CAD build for the part. Positions are in the model's coordinates, mm. Face numbers are marked on the shaded views. A direction names the side the tool comes from. Give positions to 0.01 mm unless a question says otherwise; leave off trailing zeros. Write each loop counter-clockwise with the first axis right and the second up, starting at its lowest first coordinate (ties: lowest second). Pieces come first, ordered by that corner, then holes. Notation, with made-up numbers: (-8, 51.5) - (0, 51.5) arc R35 cw to (0, 84.5) - close; hole circle Ø8 at (82.25, 52.25). An arc over 180 degrees is marked (long way). Answer as a JSON object with one key per item and string values.
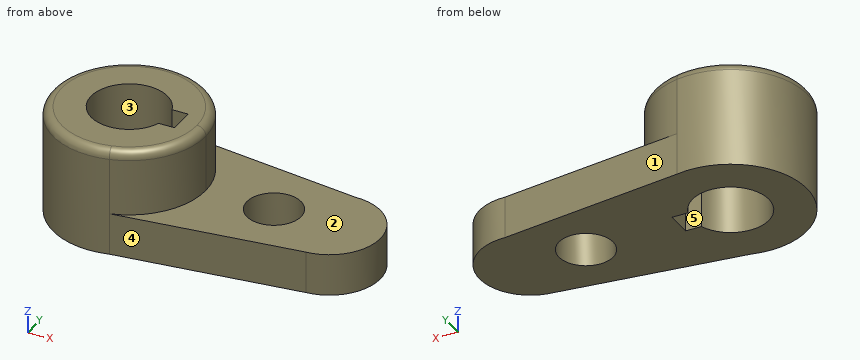
from build123d import *

# Parameters (mm, degrees)
F1_DEPTH = 15.7734
F2_DEPTH = 40.2336
F3_R     = 3.302


with BuildPart() as f1:
    # F0 (on Top) → F1 (new body)
    with BuildSketch(Plane.XY):
        with BuildLine():
            ThreePointArc((-34.39037, 28.049673), (-17.794691, 18.17528), (-11.269403, 0))
            ThreePointArc((-11.269403, 0), (-17.313196, -17.57485), (-32.887976, -27.715316))
            Line((-32.887976, -27.715316), (35.899774, -19.02012))
            ThreePointArc((35.899774, -19.02012), (53.871128, 0.678817), (34.542421, 19.04778))
            Line((34.542421, 19.04778), (-34.39037, 28.049673))
        make_face()
        with BuildLine():
            ThreePointArc((24.290597, 0), (14.130597, -10.16), (3.970597, 0))
            ThreePointArc((3.970597, 0), (14.130597, 10.16), (24.290597, 0))
        make_face(mode=Mode.SUBTRACT)
    extrude(amount=F1_DEPTH)

    # F0 (on Top) → F2 (join)
    with BuildSketch(Plane.XY):
        with BuildLine():
            ThreePointArc((-32.887976, -27.715316), (-17.313196, -17.57485), (-11.269403, 0))
            ThreePointArc((-11.269403, 0), (-17.794691, 18.17528), (-34.39037, 28.049673))
            ThreePointArc((-34.39037, 28.049673), (-68.409038, -0.769575), (-32.887976, -27.715316))
        make_face()
        with BuildLine():
            Line((-20.475368, 4.826), (-20.475368, 0))
            Line((-20.475368, 0), (-20.475368, -4.826))
            Line((-20.475368, -4.826), (-26.396638, -4.826))
            ThreePointArc((-26.396638, -4.826), (-54.131903, 0), (-26.396638, 4.826))
            Line((-26.396638, 4.826), (-20.475368, 4.826))
        make_face(mode=Mode.SUBTRACT)
    extrude(amount=F2_DEPTH)

    # F3
    f3_edges = [f1.edges().sort_by_distance(p)[0] for p in [
        (-46.80083, 27.715316, 40.2336),
    ]]
    fillet(f3_edges, radius=F3_R)


solid = f1.part
(1) 3-axis set-ups, long thin cutter, end or side, ignore diameter. For the marked faces 4 and 5: which of +Z, -Z, +X, -X, +Y, -Y reach the whole face in a straight line?
Answer key:
{"face 4": "+Z, -Z, +X, -Y", "face 5": "+Z, -Z"}
(2) Saw through at D-D, the plane x = 26. Give the cut face in (y, z), and give its area (3 significant figures).
Answer key:
{"outline": "(-20.27, 0) - (20.16, 0) - (20.16, 15.77) - (-20.27, 15.77) - close", "area": "638 mm²"}
(3) Probe L1, parallel to X at y = 6.5, z = 2; L2, parallel to X at y = 0, z = 29.5; L3, parallel to Z at x = -6, y = -0.5. List the from-to ranges inside material, lowest first. Write a range as [from, to].
Answer key:
{"L1": "x = [-67.67, -52.57], [-27.12, 6.32], [21.94, 52.74]", "L2": "x = [-68.42, -54.13], [-20.48, -11.27]", "L3": "z = [0, 15.77]"}
(4) Pull direction X, two halves, no side cores. Call the marked faces 1, 2 and 3: pulls with the +X half, pulls with the -X half, needs draft (parallel to the pull), parting line crosses it, or undercut.
Answer key:
{"face 1": "pulls with the +X half", "face 2": "needs draft", "face 3": "undercut"}
(5) Flat gauge pins, fed straight in: P1, Ø1, axis at x = -38, y = 12, coming from the +Z side; P2, Ø4.5, axis at x = -24.5, z = 16, coming from the -Y side; P3, Ø3, axis at y = 6, z = 14.5, coming from the +X side; P4, Ø1.8, axis at x = -24, z = 16, coming from the +Y side. Where does each tip first touch, or does it go through?
Answer key:
{"P1": "passes through", "P2": "stops at y = -26.94", "P3": "stops at x = 53.34", "P4": "stops at y = 26.81"}
(6) Saw through at A-A, the plane z = 8. State how many separate pieces and enclosed holes the cut face has, and give its area (3 significant figures).
Answer key:
{"separate pieces": "1", "enclosed holes": "2", "area": "4,400 mm²"}
